Design review of the part shown in the three views and the two pictorial views. Dimensions are in mm from the part's minimum x, y and z. Give positions to 0.01 mm unless a question says otherwise; leave off trailing zeros. Write each loop counter-clockwise with the first axis right and the second up, starting at its lowest first coordinate (ties: lowest second). Pieces come first, ordered by that corner, then holes.
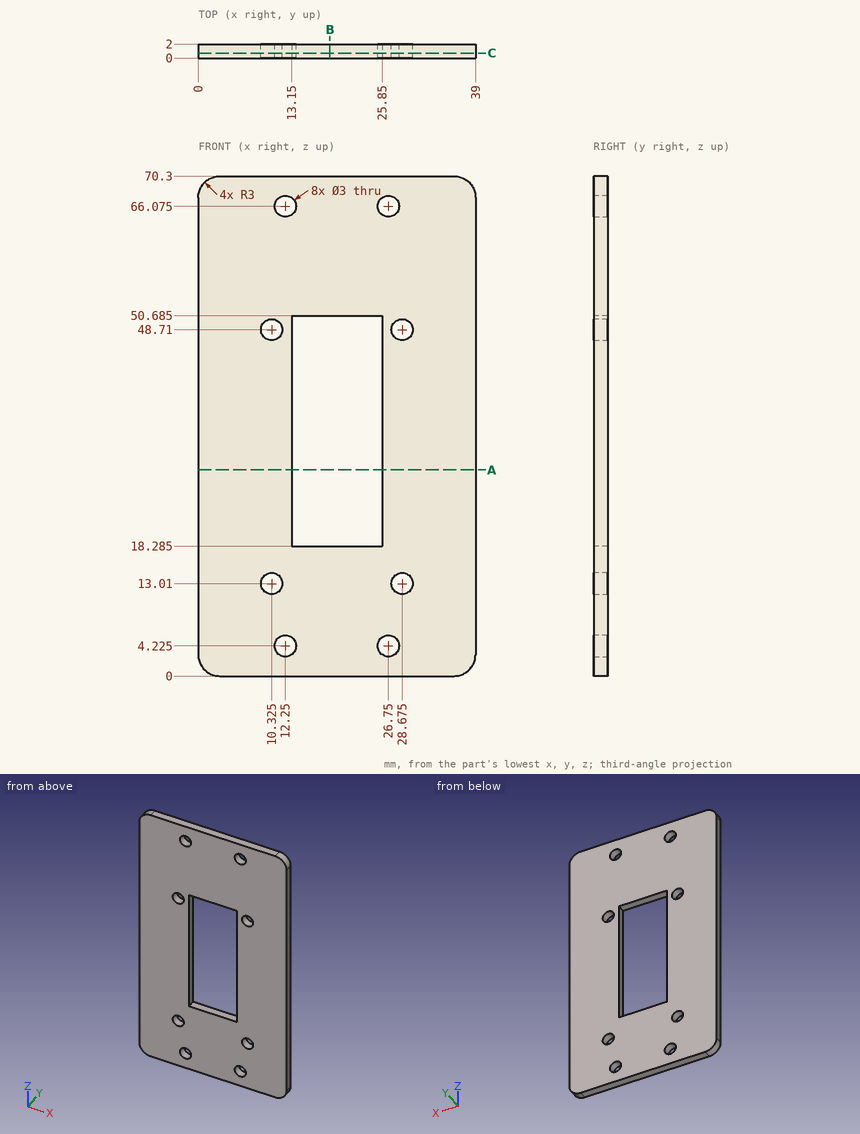
(1) Consider section C-C, the plane y = 0.7. Give the number of separate pieces and of enclosed holes in the cut face, then the cut area to 3 significant figures.
Resolved:
separate pieces: 1
enclosed holes: 9
area: 2,270 mm2
(2) Consider section A-A, the plane z = 29. Give the boundary of the cut face in (x, y), then the cut area to 3 significant figures.
Resolved:
outline: (0, 0) - (13.15, 0) - (13.15, 2) - (0, 2) - close; (25.85, 0) - (39, 0) - (39, 2) - (25.85, 2) - close
area: 52.6 mm2
(3) Clearance check with a flat-ended pin moving along its axis: P1, Ø1.8, axis at x = 10.32, z = 13.01, coming from the +Y side. State where the tip first meets the part, or that it passes through.
Resolved:
P1: passes through
(4) Consider section B-B, the plane x = 18.5. Give the boundary of the cut face in (y, z) (1 decimal).
Resolved:
outline: (0, 0) - (2, 0) - (2, 18.3) - (0, 18.3) - close; (0, 50.7) - (2, 50.7) - (2, 70.3) - (0, 70.3) - close
(5) To check wall thickness, follow L1, parallel to Z at x = 16, y = 0.95 (1 decimal); L2, parallel to X at y = 1.4, z = 34; L3, parallel to Z at x = 36.5, y = 1.35. State the ranges of each line that lie inside material, in increasing order.
Resolved:
L1: z = 0 to 18.3, 50.7 to 70.3
L2: x = 0 to 13.15, 25.85 to 39
L3: z = 0.04 to 70.26
